Model file for the job. Use its own axes, mm. Face numbers are marked on the shaded views. A direction names the side the tool comes from. Give positions to 0.01 mm unless a question says otherwise; leave off trailing zeros. Loops run counter-clockwise (first coordinate to the right, second up) from the corner with the lowest first, then second, coordinate; pieces in that order, holes last. Notation, with made-up numbers: M 41.5,54.5 L 82.5,54.5 A19 cw 82.5,91.5 Z; hole C 65,54.25 d11. An arc over 180 degrees is marked long. Answer in a Markdown table with one row per item.
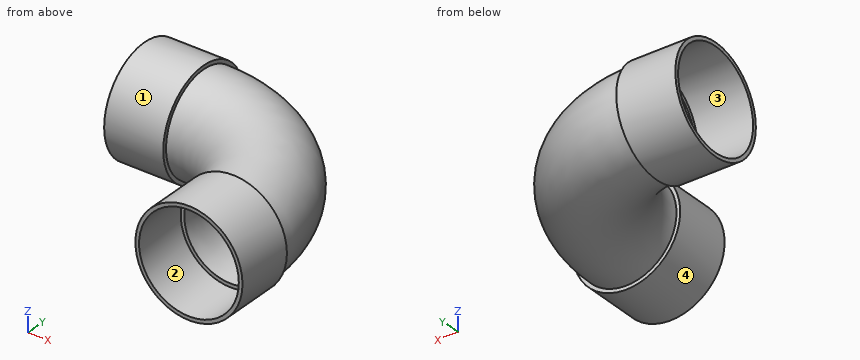
```python
from build123d import *

# Parameters (mm, degrees)
F2_R     = 27
F4_R     = 29
F4_R_2   = 27
F5_DEPTH = 32
F6_R     = 29
F6_R_2   = 27
F7_DEPTH = 32
F8_T     = -2


with BuildPart() as f3:
    # F3: sweep along a path in F0
    with BuildLine(Plane.XY) as f3_path:
        Line((-32, 65), (0, 65))
        ThreePointArc((0, 65), (45.9619407771, 45.9619407771), (65, 0))
        Line((65, 0), (65, -32))
    # F2 (on plane+point) → F3 (sweep)
    with BuildSketch(Plane.YZ.offset(-32)):
        with Locations((65, 0)):
            Circle(F2_R)
    sweep(path=f3_path.line)

    # F4 (on face) → F5 (join)
    with BuildSketch(Plane(origin=(-32, 0, 0), x_dir=(0, -1, 0), z_dir=(-1, 0, 0))):
        with Locations((-65, 0)):
            Circle(F4_R)
        with Locations((-65, 0)):
            Circle(F4_R_2, mode=Mode.SUBTRACT)
    extrude(amount=-F5_DEPTH)

    # F6 (on face) → F7 (join)
    with BuildSketch(Plane.XZ.offset(32)):
        with Locations((65, 0)):
            Circle(F6_R)
        with Locations((65, 0)):
            Circle(F6_R_2, mode=Mode.SUBTRACT)
        with Locations((65, 0)):
            Circle(F6_R_2)
    extrude(amount=-F7_DEPTH)

    # F8
    f8_openings = [f3.faces().sort_by_distance(p)[0] for p in [
        (65, -32, 0),
        (-32, 65, 0),
    ]]
    offset(amount=F8_T, openings=f8_openings, kind=Kind.INTERSECTION)


solid = f3.part
```
(1) Which spindle directions (+Z, -Z, +X, -X, +Y, -Y) get a long thin tool onto all of the face, cutting with end or side? Do the marked faces 1 and 2. Say none if no direction does.
Established:
| item | result |
|---|---|
| face 1 | -X |
| face 2 | -Y |
(2) Saw through at B-B, the plane y = -14. Give the cut face in (x, z), and give its area (3 significant figures).
Established:
| item | result |
|---|---|
| outline | C 65,0 d58; hole C 65,0 d54 |
| area | 352 mm2 |
(3) Saw through at A-A, the plane z = -20. Give the cut face in (x, y) (3 decimals), and give its area (3 significant figures).
Established:
| item | result |
|---|---|
| outline | M -32,44 L 0,44 L 0,46.862 A46.862 cw 46.862,0 L 44,0 L 44,-32 L 46.862,-32 L 46.862,-2 L 49.96,-2 A50 ccw -2,49.96 L -2,46.862 L -32,46.862 Z; M -32,83.138 L -2,83.138 L -2,79.975 A80 cw 79.975,-2 L 83.138,-2 L 83.138,-32 L 86,-32 L 86,0 L 83.138,0 A83.138 ccw 0,83.138 L 0,86 L -32,86 Z |
| area | 1,030 mm2 |
(4) Wall check: L1, parallel to Z at x = 65, y = -11.5; L2, parallel to Y at x = 27, z = -12; L3, parallel to Z at x = 42, y = 18. Give the ranges that are in metal, low to high.
Established:
| item | result |
|---|---|
| L1 | z = -29 to -27, 27 to 29 |
| L2 | y = 30.61 to 33.55, 82.63 to 85 |
| L3 | z = -18.88 to -15.88, 15.88 to 18.88 |
(5) Mould opens along Z. For the marked faces 3 and 4 say: pulls with the +Z half, pulls with the -Z half, needs draft (parallel to the pull), parting line crosses it, or undercut.
Established:
| item | result |
|---|---|
| face 3 | undercut |
| face 4 | parting line crosses it |
(6) Saw through at C-C, the plane z = 7. Give the cut face in (x, y), and give its area (3 significant figures).
Established:
| item | result |
|---|---|
| outline | M -32,36.86 L 0,36.86 L 0,38.92 A38.92 cw 38.92,0 L 36.86,0 L 36.86,-32 L 38.92,-32 L 38.92,-2 L 40.95,-2 A41 ccw -2,40.95 L -2,38.92 L -32,38.92 Z; M -32,91.08 L -2,91.08 L -2,88.98 A89 cw 88.98,-2 L 91.08,-2 L 91.08,-32 L 93.14,-32 L 93.14,0 L 91.08,0 A91.08 ccw 0,91.08 L 0,93.14 L -32,93.14 Z |
| area | 705 mm2 |
(7) Flat gauge pins, fed straight in: P1, Ø2, axis at y = 67, z = -7.5, coming from the -X side; P2, Ø3, axis at x = -17.5, y = 59, coming from the +Z side; P3, Ø4, axis at x = 49, z = -10.5, coming from the +Y side. Where does each tip first touch, or does it go through?
Established:
| item | result |
|---|---|
| P1 | stops at x = 57.08 |
| P2 | stops at z = 28.65 |
| P3 | stops at y = 76.92 |
